```python
from build123d import *

# Parameters (mm, degrees)
SALIENTE_EXTRUIR1_DEPTH = 3
SALIENTE_EXTRUIR2_DEPTH = 9.75
CROQUIS4_R              = 1.625
CORTAR_EXTRUIR1_DEPTH   = 5
CORTAR_EXTRUIR2_DEPTH   = 2
CROQUIS6_R              = 1.625
CORTAR_EXTRUIR3_DEPTH   = 9
CORTAR_EXTRUIR4_DEPTH   = 10
CROQUIS10_R             = 1.625
SALIENTE_EXTRUIR3_DEPTH = 2
CORTAR_EXTRUIR5_DEPTH   = 5
CROQUIS14_R             = 1.625
SALIENTE_EXTRUIR4_DEPTH = 3
CROQUIS15_R             = 1.625
CORTAR_EXTRUIR6_DEPTH   = 4
CORTAR_EXTRUIR7_DEPTH   = 2
CROQUIS17_R             = 1.625
CORTAR_EXTRUIR9_DEPTH   = 4
CORTAR_EXTRUIR10_DEPTH  = 2


with BuildPart() as part:
    # Croquis1 → Saliente-Extruir1 (new body)
    with BuildSketch(Plane.XY):
        with BuildLine():
            Line((-46.67593732, 50.511923567), (-55.699999998, 14.642073221))
            Line((-55.699999998, 14.642073221), (-72.78319995, 0))
            Line((-72.78319995, 0), (0, 0))
            Line((0, 0), (0, 0.68070798))
            ThreePointArc((0, 0.68070798), (-6.381456753, 18.806597842), (3.562657036, 35.25))
            Line((3.562657036, 35.25), (8.913300435, 38.25))
            Line((8.913300435, 38.25), (35.562657036, 38.25))
            Line((35.562657036, 38.25), (35.562657036, 50.511923567))
            Line((35.562657036, 50.511923567), (-46.67593732, 50.511923567))
        make_face()
    extrude(amount=-SALIENTE_EXTRUIR1_DEPTH)

    # Croquis2 → Saliente-Extruir2 (add)
    with BuildSketch(Plane(origin=(0, 0, -3), x_dir=(-1, 0, 0), z_dir=(0, 0, -1))):
        with BuildLine():
            Line((42.526447804, 46.511923567), (51.238983488, 11.880365447))
            Line((51.238983488, 11.880365447), (59.266443595, 5))
            Line((59.266443595, 5), (3.339079606, 5))
            ThreePointArc((3.339079606, 5), (1.801031086, 2.738703104), (0, 0.68070798))
            Line((0, 0.68070798), (0, 0))
            Line((0, 0), (72.78319995, 0))
            Line((72.78319995, 0), (55.699999998, 14.642073221))
            Line((55.699999998, 14.642073221), (46.67593732, 50.511923567))
            Line((46.67593732, 50.511923567), (-35.562657036, 50.511923567))
            Line((-35.562657036, 50.511923567), (-35.562657036, 38.25))
            Line((-35.562657036, 38.25), (-31.562657036, 38.25))
            Line((-31.562657036, 38.25), (-31.562657036, 46.511923567))
            Line((-31.562657036, 46.511923567), (42.526447804, 46.511923567))
        make_face()
    extrude(amount=SALIENTE_EXTRUIR2_DEPTH)

    # Croquis4 → Cortar-Extruir1 (cut)
    with BuildSketch(Plane.XZ):
        with Locations((-6.999999998, -7)):
            Circle(CROQUIS4_R)
        with Locations((-52.78319995, -7)):
            Circle(CROQUIS4_R)
    extrude(amount=-CORTAR_EXTRUIR1_DEPTH, mode=Mode.SUBTRACT)

    # Croquis5 → Cortar-Extruir2 (cut)
    with BuildSketch(Plane(origin=(0, 5, 0), x_dir=(1, 0, 0), z_dir=(0, 1, 0))):
        Polygon((-10.179999998, 7), (-8.589999998, 4.246039216), (-5.409999998, 4.246039216), (-3.819999998, 7), (-5.409999998, 9.753960784), (-8.589999998, 9.753960784), align=None)
        Polygon((-49.60319995, 7), (-51.19319995, 9.753960784), (-54.37319995, 9.753960784), (-55.96319995, 7), (-54.37319995, 4.246039216), (-51.19319995, 4.246039216), align=None)
    extrude(amount=-CORTAR_EXTRUIR2_DEPTH, mode=Mode.SUBTRACT)

    # Croquis6 → Cortar-Extruir3 (cut)
    with BuildSketch(Plane(origin=(-30.824200619, 35.963211942, 0), x_dir=(0.759271307, 0.650774217, 0), z_dir=(-0.650774217, 0.759271307, 0))):
        with Locations((-47.262195378, 6.375)):
            Circle(CROQUIS6_R)
    extrude(amount=-CORTAR_EXTRUIR3_DEPTH, mode=Mode.SUBTRACT)

    # Croquis9 → Cortar-Extruir4 (cut)
    with BuildSketch(Plane(origin=(-30.824200619, 35.963211942, 0), x_dir=(0.759271307, 0.650774217, 0), z_dir=(-0.650774217, 0.759271307, 0))):
        Polygon((-50.432195378, 6.375), (-48.847195378, 3.62969947), (-45.677195378, 3.62969947), (-44.092195378, 6.375), (-45.677195378, 9.12030053), (-48.847195378, 9.12030053), align=None)
    extrude(amount=-CORTAR_EXTRUIR4_DEPTH, mode=Mode.SUBTRACT)

    # Croquis10 → Saliente-Extruir3 (add)
    with BuildSketch(Plane(origin=(-30.824200619, 35.963211942, 0), x_dir=(0.759271307, 0.650774217, 0), z_dir=(-0.650774217, 0.759271307, 0))):
        Polygon((-50.432195378, 6.375), (-48.847195378, 3.62969947), (-45.677195378, 3.62969947), (-44.092195378, 6.375), (-45.677195378, 9.12030053), (-48.847195378, 9.12030053), align=None)
        with Locations((-47.262195378, 6.375)):
            Circle(CROQUIS10_R, mode=Mode.SUBTRACT)
    extrude(amount=-SALIENTE_EXTRUIR3_DEPTH)

    # Croquis13 → Cortar-Extruir5 (cut)
    with BuildSketch(Plane(origin=(-55.848866467, 14.050342186, 0), x_dir=(0, 0, 1), z_dir=(-0.969781373, 0.24397559, 0))):
        Polygon((-6.375, 20.547396855), (-3.621039216, 22.137396855), (-3.621039216, 25.317396855), (-6.375, 26.907396855), (-9.128960784, 25.317396855), (-9.128960784, 22.137396855), align=None)
    extrude(amount=-CORTAR_EXTRUIR5_DEPTH, mode=Mode.SUBTRACT)

    # Croquis14 → Saliente-Extruir4 (add)
    with BuildSketch(Plane(origin=(-55.848866467, 14.050342186, 0), x_dir=(0, 0, 1), z_dir=(-0.969781373, 0.24397559, 0))):
        Polygon((-6.375, 26.907396855), (-9.128960784, 25.317396855), (-9.128960784, 22.137396855), (-6.375, 20.547396855), (-3.621039216, 22.137396855), (-3.621039216, 25.317396855), align=None)
        with Locations((-6.375, 23.727396855)):
            Circle(CROQUIS14_R, mode=Mode.SUBTRACT)
    extrude(amount=-SALIENTE_EXTRUIR4_DEPTH)

    # Croquis15 → Cortar-Extruir6 (cut)
    with BuildSketch(Plane(origin=(0, 50.511923567, 0), x_dir=(1, 0, 0), z_dir=(0, 1, 0))):
        with Locations((25.562657036, 6.375)):
            Circle(CROQUIS15_R)
        with Locations((-24.437342964, 6.375)):
            Circle(CROQUIS15_R)
    extrude(amount=-CORTAR_EXTRUIR6_DEPTH, mode=Mode.SUBTRACT)

    # Croquis16 → Cortar-Extruir7 (cut)
    with BuildSketch(Plane.XZ.offset(-46.511923567)):
        Polygon((22.382657036, -6.375), (23.972657036, -9.128960784), (27.152657036, -9.128960784), (28.742657036, -6.375), (27.152657036, -3.621039216), (23.972657036, -3.621039216), align=None)
        Polygon((-21.257342964, -6.375), (-22.847342964, -3.621039216), (-26.027342964, -3.621039216), (-27.617342964, -6.375), (-26.027342964, -9.128960784), (-22.847342964, -9.128960784), align=None)
    extrude(amount=-CORTAR_EXTRUIR7_DEPTH, mode=Mode.SUBTRACT)

    # Croquis17 → Cortar-Extruir9 (cut)
    with BuildSketch(Plane(origin=(35.562657036, 0, 0), x_dir=(0, 0, -1), z_dir=(1, 0, 0))):
        with Locations((7.777494034, 42.38)):
            Circle(CROQUIS17_R)
    extrude(amount=-CORTAR_EXTRUIR9_DEPTH, mode=Mode.SUBTRACT)

    # Croquis18 → Cortar-Extruir10 (cut)
    with BuildSketch(Plane.ZY.offset(-31.562657036)):
        Polygon((-7.777494034, 39.2), (-5.02353325, 40.79), (-5.02353325, 43.97), (-7.777494034, 45.56), (-10.531454818, 43.97), (-10.531454818, 40.79), align=None)
    extrude(amount=-CORTAR_EXTRUIR10_DEPTH, mode=Mode.SUBTRACT)


solid = part.part
```
Model file for the job. Use its own axes, mm. A direction names the side the tool comes from. Give positions to 0.01 mm unless a question says otherwise; leave off trailing zeros. Order: outer loops, then holes, each group sorted by start corner. A loop starts at its lowest first (then second) coordinate and runs counter-clockwise, first axis right, second up.
1) Wall check: probe 1 along X at (y, z) = (3.5, -8); probe 2 along Z at (x, y) = (-25.5, 38.5); probe 3 along Y at (x, z) = (-56.5, -12). Give the ranges that are in metal, low to high.
2) Saw through at A-A, the plane x = -15. Write the cut outline in (y, z).
3) Saw through at D-D, the plane x = -1.5. Write the cut outline in (y, z), then the cut area to 3 significant figures.
4) 3-axis set-ups, long thin cutter, end or side, ignore diameter. For faces 1 (the flat face through (33, 42, -10.531)), 2 (the flat face through (27.96, 47.5, -5.02)), 3 (the flat face through (-5, 46.512, -8)): which of +Z, -Z, +X, -X, +Y, -Y reach the whole face in a straight line?
5) Saw through at B-B, the plane z = -11.5. Write the cut outline in (x, y), then the cut area to 3 significant figures.
6) Saw through at C-C, the plane y = 42.38. Write the cut outline in (x, z), then the cut area to 3 significant figures.
7) Pin check, flat tips, straight feed: pin 1 (1 mm diameter, centred on x = -7, y = 32.5, fed in from -Z); pin 2 (6.5 mm diameter, centred on x = 17, z = -3.5, fed in from -Y); pin 3 (3 mm diameter, centred on y = 20, z = -5, fed in from +X). Stop position of each tip, or through.
Computed:
1. probe 1: x = -68.7 to -65.63, -62.31 to -55.39, -50.18 to -9.6, -4.4 to -2.36
1. probe 2: z = -3 to 0
1. probe 3: y = 0 to 5, 7.37 to 13.96
2. outline: (0, -12.75) - (5, -12.75) - (5, -3) - (46.51, -3) - (46.51, -12.75) - (50.51, -12.75) - (50.51, 0) - (0, 0) - close
3. outline: (0, -12.75) - (2.36, -12.75) - (2.36, 0) - (0, 0) - close; (30.64, -3) - (46.51, -3) - (46.51, -12.75) - (50.51, -12.75) - (50.51, 0) - (30.64, 0) - close
3. area: 129 mm2
4. face 1: none
4. face 2: -Y
4. face 3: -Z
5. outline: (-72.78, 0) - (0, 0) - (0, 0.68) arc R22.5 cw to (-3.34, 5) - (-59.27, 5) - (-51.24, 11.88) - (-42.53, 46.51) - (31.56, 46.51) - (31.56, 38.25) - (35.56, 38.25) - (35.56, 50.51) - (-46.68, 50.51) - (-55.7, 14.64) - close
5. area: 940 mm2
6. outline: (-48.72, -12.75) - (-43.57, -12.75) - (-43.57, -3) - (31.56, -3) - (31.56, -5.02) - (33.56, -5.02) - (33.56, -6.15) - (35.56, -6.15) - (35.56, 0) - (-48.72, 0) - close; (31.56, -12.75) - (35.56, -12.75) - (35.56, -9.4) - (33.56, -9.4) - (33.56, -10.53) - (31.56, -10.53) - close
6. area: 325 mm2
7. pin 1: stops at z = -3
7. pin 2: stops at y = 38.25
7. pin 3: stops at x = -48.82
